The model under review builds one solid part; all positions refer to its coordinate system, in mm. A direction names the side the tool comes from. Round coordinates to 2 decimals unless told otherwise and drop trailing zeros. Loops run counter-clockwise (first coordinate to the right, second up) from the corner with the lowest first, then second, coordinate; pieces in that order, holes last. Notation, with made-up numbers: (64, -17.75) -> (81, -17.75) arc R17 cw to (81, 12.25) -> close; hole circle Ø11 at (-18.75, 79). An arc over 180 degrees is marked (long way). Return JSON: item names as keys, results as strings. Group by question number.
```python
from build123d import *

# Parameters (mm, degrees)
F_01_BASE_PROFILE_W           = 330
F_01_BASE_PROFILE_H           = 330
F_01_BASE_PROFILE_R           = 7
F_01_BASE_PROFILE_R_2         = 5.248628476
F_01_BASE_PROFILE_R_3         = 5.751371524
F_01_BASE_EXTRUDE_DEPTH       = 14
F_02_BOSS_PROFILE_R           = 105
F_02_REINFORCEMENT_BOSS_DEPTH = 22


with BuildPart() as part:
    # 01_Base_Profile → 01_Base_Extrude (new body)
    with BuildSketch(Plane(origin=(0, 0, 0), x_dir=(1, 0, 0), z_dir=(0, 1, 0))):
        Rectangle(F_01_BASE_PROFILE_W, F_01_BASE_PROFILE_H)
        with Locations(Location((120.104339226, 49.748846207, 0), (0, 0, 270))):
            Circle(F_01_BASE_PROFILE_R, mode=Mode.SUBTRACT)
        with Locations(Location((49.748846207, 120.104339226, 0), (0, 0, 270))):
            Circle(F_01_BASE_PROFILE_R, mode=Mode.SUBTRACT)
        with Locations(Location((-49.748846207, 120.104339226, 0), (0, 0, 270))):
            Circle(F_01_BASE_PROFILE_R, mode=Mode.SUBTRACT)
        with Locations(Location((-120.104339226, 49.748846207, 0), (0, 0, 270))):
            Circle(F_01_BASE_PROFILE_R, mode=Mode.SUBTRACT)
        with Locations(Location((-120.104339226, -49.748846207, 0), (0, 0, 270))):
            Circle(F_01_BASE_PROFILE_R, mode=Mode.SUBTRACT)
        with Locations(Location((-49.748846207, -120.104339226, 0), (0, 0, 270))):
            Circle(F_01_BASE_PROFILE_R, mode=Mode.SUBTRACT)
        with Locations(Location((49.748846207, -120.104339226, 0), (0, 0, 270))):
            Circle(F_01_BASE_PROFILE_R, mode=Mode.SUBTRACT)
        with Locations(Location((120.104339226, -49.748846207, 0), (0, 0, 270))):
            Circle(F_01_BASE_PROFILE_R, mode=Mode.SUBTRACT)
        with Locations(Location((49.748846207, 49.748846207, 0), (0, 0, 270))):
            Circle(F_01_BASE_PROFILE_R_2, mode=Mode.SUBTRACT)
        with Locations(Location((-49.748846207, 49.748846207, 0), (0, 0, 270))):
            Circle(F_01_BASE_PROFILE_R_3, mode=Mode.SUBTRACT)
        with Locations(Location((-49.748846207, -49.748846207, 0), (0, 0, 270))):
            Circle(F_01_BASE_PROFILE_R_3, mode=Mode.SUBTRACT)
        with Locations(Location((49.748846207, -49.748846207, 0), (0, 0, 270))):
            Circle(F_01_BASE_PROFILE_R_2, mode=Mode.SUBTRACT)
    extrude(amount=F_01_BASE_EXTRUDE_DEPTH)

    # 02_Boss_Profile → 02_Reinforcement_Boss (add)
    with BuildSketch(Plane(origin=(0, 0, 0), x_dir=(1, 0, 0), z_dir=(0, 1, 0))):
        with Locations(Location((0, 0, 0), (0, 0, 90))):
            Circle(F_02_BOSS_PROFILE_R)
    extrude(amount=F_02_REINFORCEMENT_BOSS_DEPTH)


solid = part.part
```
1. We need section A-A, the plane z = 0. Write out the cut boundary in (x, y).
2. For P1, Ø5, axis at x = -36, z = -25.5, coming from the -Y side; P2, Ø2, axis at y = 17, z = -19, coming from the -X side; P3, Ø2, axis at y = 16.5, z = -96, coming from the +X side; P4, Ø1, axis at x = 7, y = 19, coming from the +Z side, all flat-tipped, find the tip position at first contact; note any pin that passes through.
3. Draft analysis for pull direction Z (two halves, no side actions). For faces 1 (the face through (-126.938, 6.902, -51.266)), 2 (the face through (-2, 7, 165)), 3 (the face through (-76, 14, -76)), state which applies: pulls with the +Z half, pulls with the -Z half, needs draft (parallel to the pull), parting line crosses it, or undercut.
4. Wall thickness on line 1 (Y direction, x = 55, z = -145.5); line 2 (X direction, y = 3.5, z = -117.5); line 3 (Z direction, x = -95.5, y = 18): over which ranges is each line inside the solid? List them lowest first.
5. We need section C-C, the plane x = -133. Write out the cut boundary in (y, z).
6. Tool access review of faces 4 (the face through (-165, 7, 2)), 5 (the face through (-31.54, 17.94, -100.15)): name each direction out of +Z, -Z, +X, -X, +Y, -Y from which nothing blocks a thin tool from reaching the whole face with its end or side.
7. We need section B-B, the plane x = 0. Write out the cut boundary in (y, z), then the cut area to 3 significant figures.
Check sheet entries:
{
 "1": {"outline": "(-165, 0) -> (165, 0) -> (165, 14) -> (105, 14) -> (105, 22) -> (-105, 22) -> (-105, 14) -> (-165, 14) -> close"},
 "2": {"P1": "stops at y = 0", "P2": "stops at x = -103.45", "P3": "stops at x = 44.72", "P4": "stops at z = 104.8"},
 "3": {"face 1": "undercut", "face 2": "pulls with the +Z half", "face 3": "needs draft"},
 "4": {"line 1": "y = 0 to 14", "line 2": "x = -165 to -56.25, -43.25 to 43.25, 56.25 to 165", "line 3": "z = -43.64 to 43.64"},
 "5": {"outline": "(0, -165) -> (14, -165) -> (14, 165) -> (0, 165) -> close"},
 "6": {"face 4": "+Z, -Z, -X, +Y, -Y", "face 5": "+Y"},
 "7": {"outline": "(0, -165) -> (14, -165) -> (14, -105) -> (22, -105) -> (22, 105) -> (14, 105) -> (14, 165) -> (0, 165) -> close", "area": "6,300 mm²"}
}
